Read the model definition and answer for the solid it produces. Units are mm, in the model's axes. Face numbers are marked on the shaded views. A direction names the side the tool comes from. Give positions to 0.01 mm unless a question says otherwise; leave off trailing zeros. Loops run counter-clockwise (first coordinate to the right, second up) from the corner with the lowest first, then second, coordinate; pieces in that order, holes last. Notation, with made-up numbers: (45, 87.5) - (50, 87.5) arc R28 cw to (50, 120.5) - close; hole circle Ø5 at (77.5, 86). An arc over 180 degrees is marked (long way). Write each question's results on one line, items separated by ' | '. Start each with the question number.
Q1. Determine the mould class of the marked faces 1, 2 and 3 for opening direction Z: +Z half, -Z half, draft (parallel to the pull), parting line (faces both ways), or undercut.
Q2. For the marked faces 4, 5 and 6, determine the directions among +Z, -Z, +X, -X, +Y, -Y from which every point of the face is accessible in a straight line to the end or side of a thin tool.
Q3. Given pin 1 (1.5 mm diameter, centred on y = 3.5, z = 1, fed in from -X); pin 2 (3 mm diameter, centred on y = -2.5, z = 2, fed in from -X), each flat-ended and moving along its own axis, determine where each tip first touches the part or whether it passes through.
Q4. The part is cut by section B-B, the plane y = -1. Write down the section's boundary in (x, z), plus the area to 3 significant figures.
Q5. The part is cut by section A-A, the plane z = 0. Write down the section's boundary in (x, y), plus the area to 3 significant figures.
Q6. Find the intervals of material crossed by line 1 (Y direction, x = -2.2, z = 0.3); line 2 (Z direction, x = 0.05, y = 2.5); line 3 (Z direction, x = 1.55, y = 4.25), in increasing order. Write a range as from..to.
Autodesk Inventor part; units mm, degrees
ref_plane "YZ Plane" through (0, 0, 0) normal (1, 0, 0) x (0, 1, 0)
ref_plane "XZ Plane" through (0, 0, 0) normal (0, 1, 0) x (-1, 0, 0)
ref_plane "XY Plane" through (0, 0, 0) normal (0, 0, 1) x (1, 0, 0)
sketch "Sketch1" plane through (0, 0, 0) normal (0, 0, 1) x (1, 0, 0)
  line L0 (0, 4.5) -> (0, -4.5)
  line L1 (0, -4.5) -> (1.25, -4.5)
  line L2 (1.25, -4.5) -> (1.5, -4.25)
  line L3 (1.5, -4.25) -> (1.5, 3.4)
  line L4 (1.6, 3.5) -> (2.75, 3.5)
  line L5 (2.75, 3.5) -> (2.75, 4.35)
  line L6 (2.6, 4.5) -> (0, 4.5)
  arc A0 (1.6, 3.5) -> (1.5, 3.4) centre (1.6, 3.4) ccw
  line L7 (2.6, 4.5) -> (2.75, 4.35)
  point P0 (0, 0)
  point P1 (2.75, 4.5)
  point P2 (0, 0)
  dimension "d0" = 5.5
  dimension "d1" = 1
  dimension "d3" = 3
  dimension "d4" = 3.2
  dimension "d5" = 135
  dimension "d6" = 0.25
  dimension "d7" = 8
  dimension "d18" = 0.15
  dimension "d22" = 0.15
revolve "Revolution1" add sketch "Sketch1" angle 360 about axis through (0, 4.5, 0) along (0, -1, 0)
sketch "Sketch2" plane through (0, 4.5, 0) normal (0, 1, 0) x (1, 0, 0)
  line L0 (0, -1.1547) -> (-1, -0.5774)
  line L1 (-1, -0.5774) -> (-1, 0.5774)
  line L2 (-1, 0.5774) -> (0, 1.1547)
  line L3 (0, 1.1547) -> (1, 0.5774)
  line L4 (1, 0.5774) -> (1, -0.5774)
  line L5 (1, -0.5774) -> (0, -1.1547)
  point P0 (0, 0)
  point P1 (0, 0)
  dimension "d11" = 2
extrude "Extrusion1" cut sketch "Sketch2" against normal blind 1
thread "Thread1"
sketch "Sketch3" plane through (0, 0, 0) normal (1, 0, 0) x (0, 1, 0)
  line L0 (4.5, 1.1547) -> (4.5, 0.5774)
  line L1 (4.5, 1.1547) -> (4, 0.6547)
  line L2 (4, 0.6547) -> (4.5, 0.6547)
  line L3 (4.5, 0.6547) -> (4.5, 1.1547)
  line L4 (-0.9, 0) -> (5.4, 0)
  point P0 (0, 0)
  dimension "d16" = 0.5
revolve "Revolution2" cut sketch "Sketch3" angle 360 about axis through (0, -10, 0) along (0, 1, 0)
equation "\"d22\" = d18"
properties part number "Bolt_M3x0.35_6mm_SH" material "Stainless Steel"
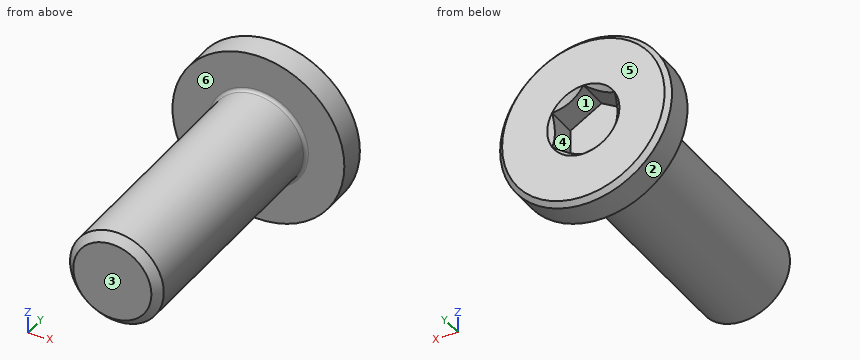
Check sheet entries:
1) face 1: undercut | face 2: parting line | face 3: draft
2) face 4: +Y | face 5: +Z, -Z, +X, -X, +Y | face 6: -Y
3) pin 1: stops at x = -2.74 | pin 2: stops at x = -1.41
4) outline: circle Ø3 at (0, 0) | area: 7.07 mm^2
5) outline: (-2.75, 3.5) - (-1.6, 3.5) arc R0.1 cw to (-1.5, 3.4) - (-1.5, -4.25) - (-1.25, -4.5) - (1.25, -4.5) - (1.5, -4.25) - (1.5, 3.4) arc R0.1 cw to (1.6, 3.5) - (2.75, 3.5) - (2.75, 4.35) - (2.6, 4.5) - (1.15, 4.5) - (1, 4.35) - (1, 3.5) - (-1, 3.5) - (-1, 4.35) - (-1.15, 4.5) - (-2.6, 4.5) - (-2.75, 4.35) - close | area: 27.4 mm^2
6) line 1: y = 3.5..4.5 | line 2: z = -1.5..1.5 | line 3: z = -2.27..2.27
